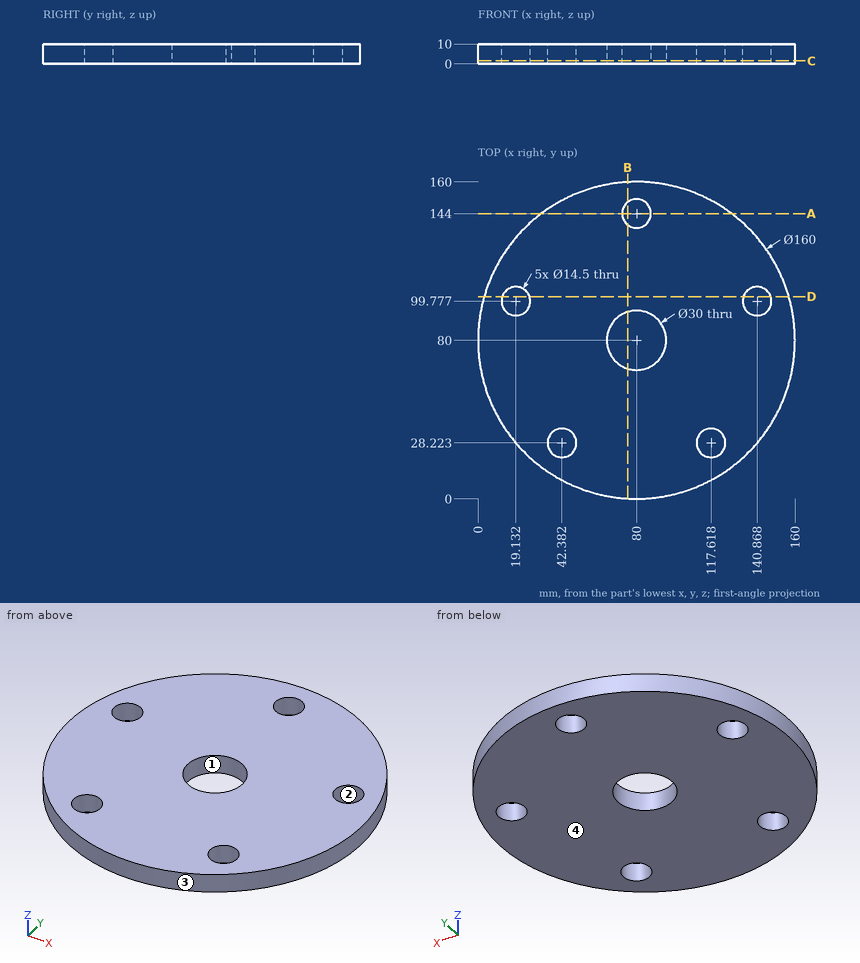
Can you work these out from the drawing? Everything is in mm from the part's minimum corner. Round coordinates to 2 decimals unless told otherwise and drop trailing zeros. Loops run counter-clockwise (first coordinate to the right, second up) from the corner with the lowest first, then second, coordinate; pieces in that order, holes last. Notation, with made-up numbers: (-24.75, -21) -> (25.25, -21) arc R29 ccw to (25.25, 0) -> close; hole circle Ø11 at (-24, -8). An arc over 180 degrees is marked (long way). One line per question, with ' | ' between items.
(1) If we section it at A-A on y = 144: List the corners of the cut face in (x, z) for me.
Model answer:
outline: (32, 0) -> (72.75, 0) -> (72.75, 10) -> (32, 10) -> close; (87.25, 0) -> (128, 0) -> (128, 10) -> (87.25, 10) -> close
(2) If we section it at D-D on y = 102: List the corners of the cut face in (x, z) for me (1 decimal).
Model answer:
outline: (3.1, 0) -> (12.2, 0) -> (12.2, 10) -> (3.1, 10) -> close; (26, 0) -> (134, 0) -> (134, 10) -> (26, 10) -> close; (147.8, 0) -> (156.9, 0) -> (156.9, 10) -> (147.8, 10) -> close
(3) If we section it at C-C on z = 1.5: Count the separate pieces of the cut face and the enclosed holes in it, and give its area (3 significant figures).
Model answer:
separate pieces: 1 | enclosed holes: 6 | area: 18,600 mm^2
(4) Thinking about a two-plate mould opening in X: for the marked faces 1, 2, 3 and 4, which applies, released by +X, released by -X, zero draft, split by the parting line, or undercut?
Model answer:
face 1: undercut | face 2: undercut | face 3: split by the parting line | face 4: zero draft
(5) If I drill on probe 1 along Y at (x, z) = (80, 7.25); probe 2 along X at (y, z) = (26, 4) (1 decimal); probe 3 along X at (y, z) = (79.5, 5), over which ranges is the centre line in solid material (lowest first)?
Model answer:
probe 1: y = 0 to 65, 95 to 136.75, 151.25 to 160 | probe 2: x = 21 to 35.5, 49.3 to 110.7, 124.5 to 139 | probe 3: x = 0 to 65.01, 94.99 to 160
(6) For pin 1 Ø11.5 at (x, y) = (140.87, 99.78) entering from -Z; pin 2 Ø2 at (y, z) = (67, 3) entering from +X (1 decimal); pin 3 Ø1 at (y, z) = (48.5, 1.5) entering from -X; pin 4 Ø1.5 at (x, z) = (136, 8.5) entering from -Y, each with a flat end and sliding along its axis, tell me the tip position at first contact or that it passes through.
Model answer:
pin 1: passes through | pin 2: stops at x = 159.1 | pin 3: stops at x = 6.25 | pin 4: stops at y = 22.14
(7) If we section it at B-B on x = 75.5: List the corners of the cut face in (y, z) for me (1 decimal), and give its area (3 significant figures).
Model answer:
outline: (0.1, 0) -> (65.7, 0) -> (65.7, 10) -> (0.1, 10) -> close; (94.3, 0) -> (138.3, 0) -> (138.3, 10) -> (94.3, 10) -> close; (149.7, 0) -> (159.9, 0) -> (159.9, 10) -> (149.7, 10) -> close | area: 1,200 mm^2
